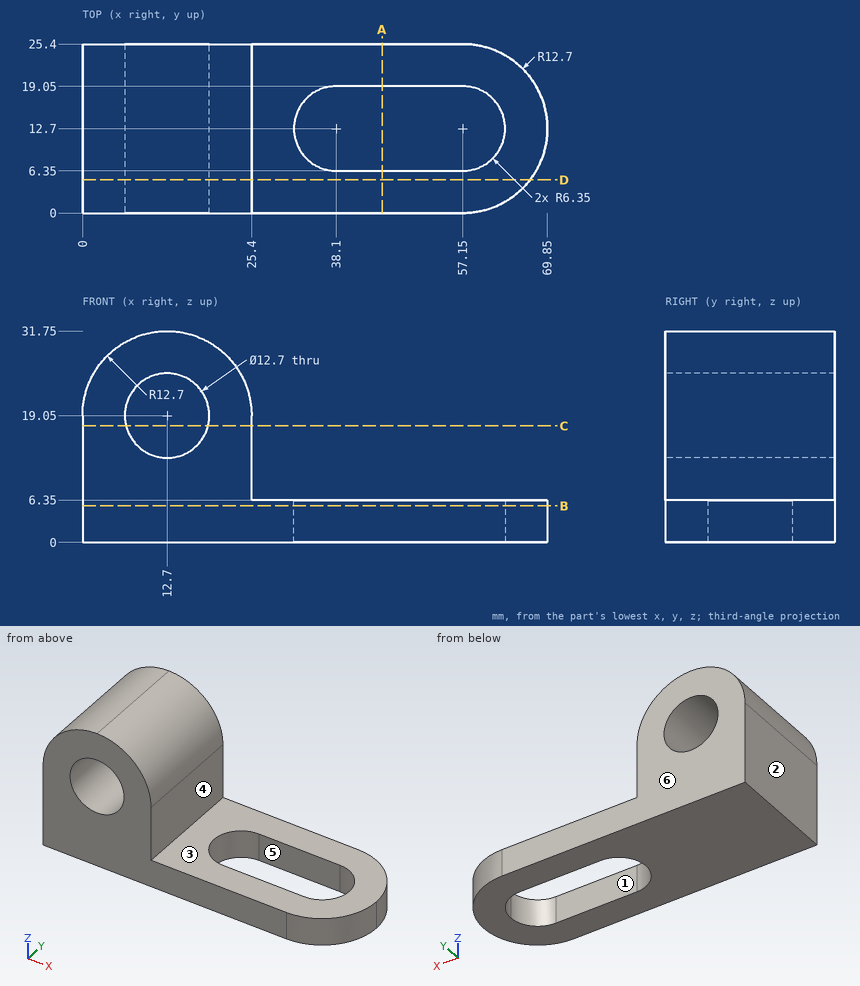
Design review of the part shown in the three views and the two pictorial views. Dimensions are in mm from the part's minimum x, y and z. A direction names the side the tool comes from. Coordinates: 2 decimals unless noted, no trailing zeros. Loops run counter-clockwise (first coordinate to the right, second up) from the corner with the lowest first, then second, coordinate; pieces in that order, holes last.
(1) Consider section D-D, the plane y = 5. Give the boundary of the cut face in (x, z), plus the area to 3 significant figures.
Determined:
outline: (0, 0) - (67.25, 0) - (67.25, 6.35) - (25.4, 6.35) - (25.4, 19.05) arc R12.7 ccw to (0, 19.05) - close; hole circle Ø12.7 at (12.7, 19.05)
area: 876 mm2
(2) Wall thickness on L1, parallel to X at y = 13.75, z = 19.5; L2, parallel to Z at x = 12.7, y = 12; L3, parallel to Z at x = 43, y = 23.5: over which ranges is each line inside the solid? List them lowest first.
Determined:
L1: x = 0.01 to 6.37, 19.03 to 25.39
L2: z = 0 to 12.7, 25.4 to 31.75
L3: z = 0 to 6.35
(3) Insertion check: P1, Ø12, axis at x = 28.5, y = 6, coming from the +Z side; P2, Ø5, axis at x = 38.5, y = 2.5, coming from the +Z side; P3, Ø1, axis at y = 7.5, z = 22, coming from the -X side; P4, Ø10, axis at y = 16, z = 9.5, coming from the +X side. Each pin has a flat end and moves straight along its axis. Give the tip position at first contact, or say it passes through.
Determined:
P1: stops at z = 27.13
P2: stops at z = 6.35
P3: stops at x = 0.24
P4: stops at x = 69.85
(4) Draft analysis for pull direction Y (two halves, no side actions). For the marked faces 4, 5 and 6, state which applies: +Y half, -Y half, draft (parallel to the pull), parting line (faces both ways), or undercut.
Determined:
face 4: draft
face 5: undercut
face 6: +Y half
(5) Consider section A-A, the plane x = 45. Give the boundary of the cut face in (y, z), plus the area to 3 significant figures.
Determined:
outline: (0, 0) - (6.35, 0) - (6.35, 6.35) - (0, 6.35) - close; (19.05, 0) - (25.4, 0) - (25.4, 6.35) - (19.05, 6.35) - close
area: 80.6 mm2
(6) Tool access review of the marked faces 1, 2 and 3: name each direction out of +Z, -Z, +X, -X, +Y, -Y from which nothing blocks a thin tool from reaching the whole face with its end or side.
Determined:
face 1: +Z, -Z
face 2: +Z, -Z, -X, +Y, -Y
face 3: +Z, +X, +Y, -Y
(7) Consider section B-B, the plane z = 5.5. Give the boundary of the cut face in (x, y).
Determined:
outline: (0, 0) - (57.15, 0) arc R12.7 ccw to (57.15, 25.4) - (0, 25.4) - close; hole (38.1, 6.35) - (57.15, 6.35) arc R6.35 ccw to (57.15, 19.05) - (38.1, 19.05) arc R6.35 ccw to start
(8) Consider section C-C, the plane z = 17.5. Give the boundary of the cut face in (x, y), plus the area to 3 significant figures.
Determined:
outline: (0, 0) - (6.54, 0) - (6.54, 25.4) - (0, 25.4) - close; (18.86, 0) - (25.4, 0) - (25.4, 25.4) - (18.86, 25.4) - close
area: 332 mm2
